Could you check a few things on this drawing? It's one solid part, dimensions in mm from its lowest x, y, z. A direction names the side the tool comes from. Give positions to 0.01 mm unless a question says otherwise; leave off trailing zeros. Loops run counter-clockwise (first coordinate to the right, second up) from the corner with the lowest first, then second, coordinate; pieces in that order, holes last. Notation, with made-up numbers: (78.5, 5.25) - (82.5, 5.25) arc R34 ccw to (82.5, 38.25) - close; hole circle Ø8 at (-34.5, -5). An arc over 180 degrees is marked (long way). Return JSON: item names as keys, results as strings. Group by question number.
(1) I need wall thicknesses on probe 1 along Z at (x, y) = (6, 32); probe 2 along Y at (x, z) = (33, 12); probe 3 along Z at (x, y) = (42, 69). Which ranges of each line are inside material? Lowest first, please. Write a range as [from, to].
(2) On a 3-axis mill with a long thin cutter (end or side, diameter ignored), from which of +Z, -Z, +X, -X, +Y, -Y can I reach the whole of each face in a straight line? I mean the marked faces 1, 2, 3, 4 and 5. Say none if no direction works.
(3) If we section it at A-A (y = 19.05): State how many separate pieces and enclosed holes the cut face has.
(4) For P1, Ø7.5, axis at y = 38, z = 13, coming from the -X side (1 decimal); P2, Ø5, axis at y = 38, z = 70, coming from the -X side; P3, Ø10, axis at x = 33, z = 49, coming from the +Y side; P4, Ø5, axis at x = 21.5, z = 85, coming from the +Y side, each with a flat end and sliding along its axis, tell me the tip position at first contact or that it passes through.
(5) If we mould it in two halves opening along Z, with no side actions, what happens to the marked faces 6, 7 and 8? For each: released by +Z, released by -Z, zero draft, split by the parting line, or undercut.
(6) If we section it at D-D (x = 9.5): Please give me the cut outline in (y, z).
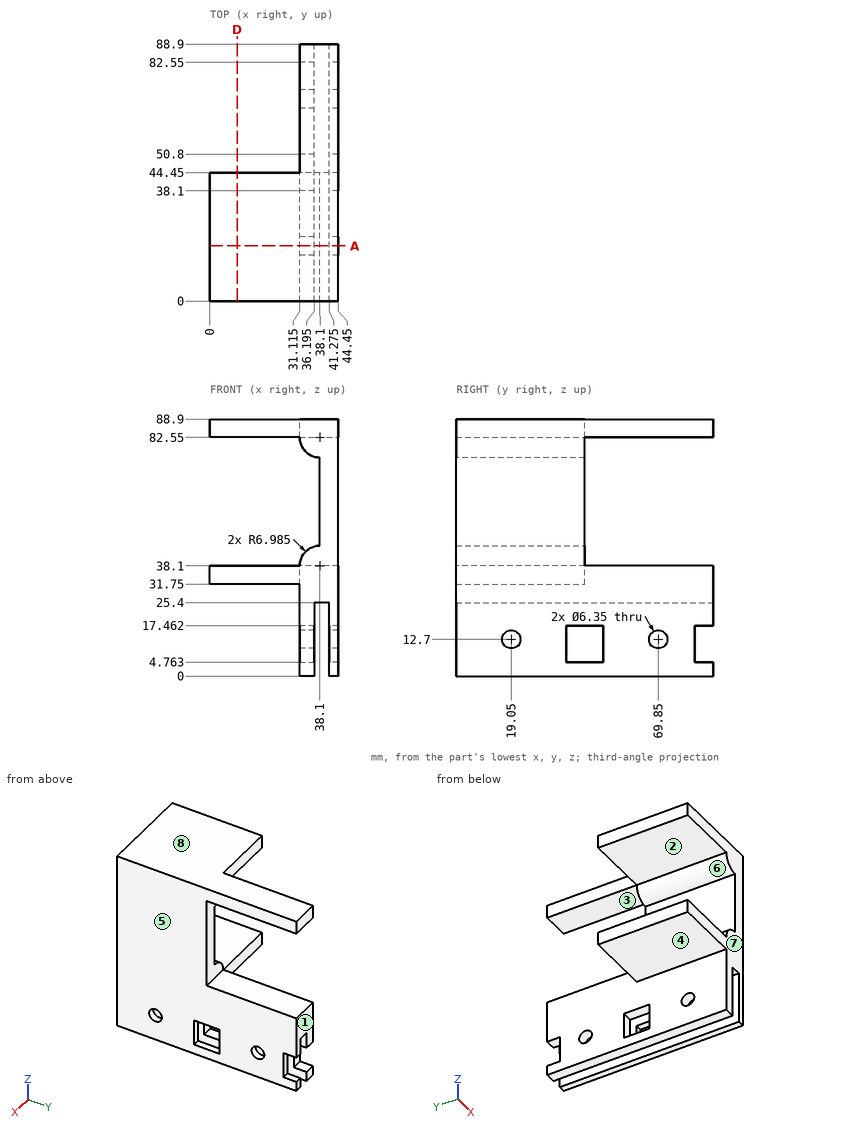
Values:
{
 "1": {"probe 1": "[31.75, 38.1], [82.55, 88.9]", "probe 2": "[0, 15.95], [22.15, 38.1], [50.8, 66.75], [72.95, 82.55]", "probe 3": "[0, 9.64], [15.76, 38.1], [82.55, 88.9]"},
 "2": {"face 1": "+Z, -Z, +X, -X, +Y", "face 2": "-X, +Y, -Y", "face 3": "+X, -X, +Y", "face 4": "-Z, -X, +Y, -Y", "face 5": "+Z, -Z, +X, +Y, -Y"},
 "3": {"separate pieces": "3", "enclosed holes": "0"},
 "4": {"P1": "x = 31.1", "P2": "x = 38.1", "P3": "through", "P4": "y = 44.45"},
 "5": {"face 6": "undercut", "face 7": "zero draft", "face 8": "released by +Z"},
 "6": {"outline": "(0, 31.75) - (44.45, 31.75) - (44.45, 38.1) - (0, 38.1) - close; (0, 82.55) - (44.45, 82.55) - (44.45, 88.9) - (0, 88.9) - close"}
}
